Check sheet for the modelled part. Datum: model origin and axes. Units: mm. Face numbers are marked on the shaded views. Give positions to 0.01 mm unless a question says otherwise; leave off trailing zeros. Answer in a Markdown table with one row per item. Add a question column.
(1) Draft check along X on the marked faces 1 and 2. Enter one of: released by +X, released by -X, zero draft, split by the parting line, or undercut.
(2) Thickness scan on L1, parallel to Z at x = 10.5, y = 10; L2, parallel to Y at x = 0, z = 2.55; L3, parallel to Y at x = 0, z = 2.1. Record the ranges inside material, lowest first.
(3) Go/stop test with flat-tipped pins: P1, Ø2, axis at x = -22.5, y = -5, coming from the +Z side; P2, Ø1.5, axis at y = -7, z = 4.5, coming from the +X side; P3, Ø3, axis at y = 21.5, z = 7.5, coming from the -X side. Record where each tip stops, or that it passes through.
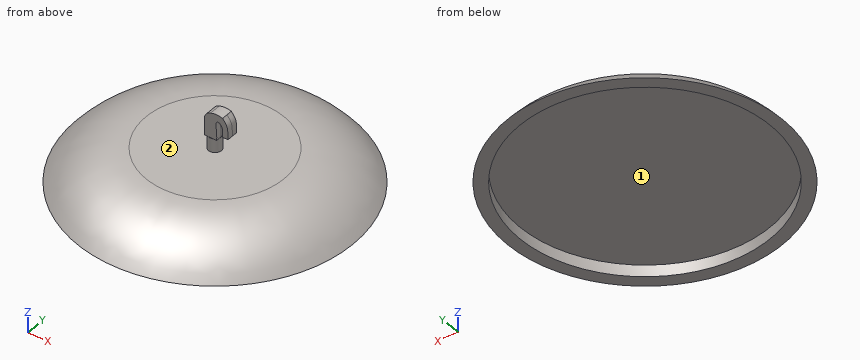
from build123d import *

# Parameters (mm, degrees)
F0_R     = 50.8
F1_DEPTH = 12.7
F4_R     = 2.3844019002
F5_DEPTH = 5.08
F7_DEPTH = 2.159
F8_R     = 46.183577677
F9_DEPTH = 4.318


# Not quite as in the source:
# - a fillet or chamfer that OpenCascade refuses, or shapes differently, is made with other operations: its cross-section is extruded or revolved along the edge and cut away or added


with BuildPart() as f1:
    # F0 (on Top) → F1 (new body)
    with BuildSketch(Plane.XY):
        Circle(F0_R)
    extrude(amount=F1_DEPTH)

    # F2: fillet of radius 31.75 on 1 edges, made by hand

    # F2_s1 → F2_t2 (revolve, cut)
    with BuildSketch(Plane.XZ):
        with BuildLine():
            ThreePointArc((50.8, 0), (39.5990316571, 9.3480633142), (25.4, 12.7))
            Line((25.4, 12.7), (50.8, 12.7))
            Line((50.8, 12.7), (50.8, 0))
        make_face()
    revolve(axis=Axis((0, 0, 12.7), (0, 0, 1)), mode=Mode.SUBTRACT)

    # F4 (on face) → F5 (join)
    with BuildSketch(Plane.XY.offset(12.7)):
        Circle(F4_R)
    extrude(amount=F5_DEPTH)

    # F6 (on Front) → F7 (join, symmetric)
    with BuildSketch(Plane.XZ):
        with BuildLine():
            Line((-2.3349747062, 23.7907841802), (-2.3349747062, 17.8023930639))
            Line((-2.3349747062, 17.8023930639), (2.1964372136, 17.6963582635))
            add(Edge.make_bspline(
                [(4.347205162, 19.8880601674), (4.4335474069, 20.8885193067), (4.5909606666, 22.7124852177), (3.6400970731, 24.6070794631), (1.4756871927, 24.9554852281), (2.3553322785, 19.8781417965), (2.2437732053, 18.3463361327), (2.1964372136, 17.6963582635)],
                knots=[0, 0, 0, 0, 0.2170343083, 0.395681564, 0.5347797532, 0.8025976366, 1, 1, 1, 1], degree=3))
            Line((4.347205162, 19.8880601674), (6.3592605293, 19.8880601674))
            add(Edge.make_bspline(
                [(4.3928744271, 26.9053261727), (5.0263463985, 26.1760936525), (6.4510931733, 24.5359710236), (6.3920513007, 21.5476896096), (6.3592605293, 19.8880601674)],
                knots=[0, 0, 0, 0, 0.4446207541, 1, 1, 1, 1], degree=3))
            ThreePointArc((4.3928744271, 26.9053261727), (2.1964372136, 27.2497590183), (0, 26.9053261727))
            ThreePointArc((0, 26.9053261727), (-1.6864120154, 25.7370934247), (-2.3349747062, 23.7907841802))
        make_face()
    extrude(amount=F7_DEPTH, both=True)

    # F8 (on face) → F9 (cut)
    with BuildSketch(Plane(origin=(0, 0, 0), x_dir=(1, 0, 0), z_dir=(0, 0, -1))):
        Circle(F8_R)
    extrude(amount=-F9_DEPTH, mode=Mode.SUBTRACT)


solid = f1.part
Reply:
| question | item | result |
|---|---|---|
| 1 | face 1 | undercut |
| 1 | face 2 | zero draft |
| 2 | L1 | 4.32 to 12.7 |
| 2 | L2 | -48.67 to -46.18, 46.18 to 48.67 |
| 2 | L3 | -49.08 to -46.18, 46.18 to 49.08 |
| 3 | P1 | z = 12.7 |
| 3 | P2 | x = 46.98 |
| 3 | P3 | x = -39.57 |
